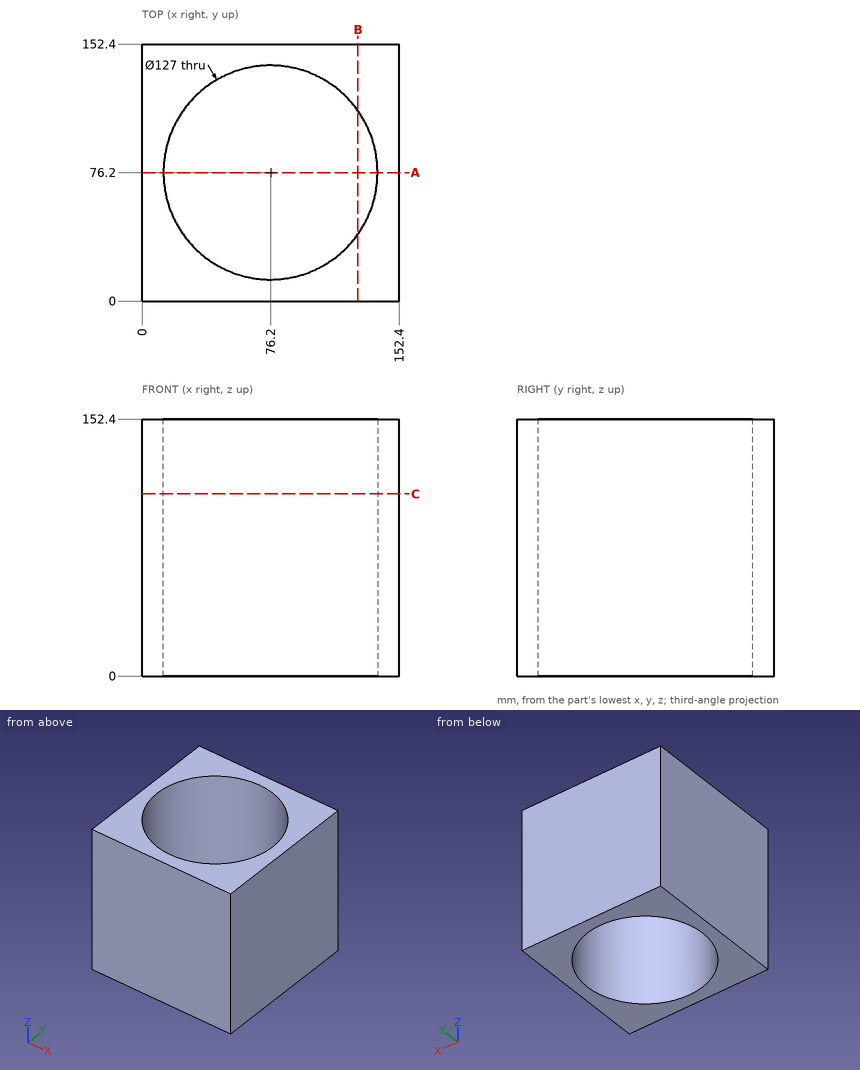
Design review of the part shown in the three views and the two pictorial views. Dimensions are in mm from the part's minimum x, y and z. Coordinates: 2 decimals unless noted, no trailing zeros. Loops run counter-clockwise (first coordinate to the right, second up) from the corner with the lowest first, then second, coordinate; pieces in that order, holes last. Notation, with made-up numbers: M -13.75,25 L 35.25,25 A22 ccw 35.25,37 Z; hole C 62.25,42.25 d7. An arc over 180 degrees is marked long. Put each result on its own line as item: value. Start each with the question number.
Q1. Add section B-B (x = 128). Write out the cut boundary in (y, z).
Q2. Wall thickness on line 1 (X direction, y = 76, z = 45); line 2 (Y direction, x = 130.5, z = 123.5): over which ranges is each line inside the solid? List them lowest first.
Q3. Add section A-A (y = 76.2). Write out the cut boundary in (x, z), and give its area (3 significant figures).
Q4. Add section C-C (z = 108). Write out the cut boundary in (x, y).
Answers:
1. outline: M 0,0 L 39.47,0 L 39.47,152.4 L 0,152.4 Z; M 112.93,0 L 152.4,0 L 152.4,152.4 L 112.93,152.4 Z
2. line 1: x = 0 to 12.7, 139.7 to 152.4
2. line 2: y = 0 to 43.28, 109.12 to 152.4
3. outline: M 0,0 L 12.7,0 L 12.7,152.4 L 0,152.4 Z; M 139.7,0 L 152.4,0 L 152.4,152.4 L 139.7,152.4 Z
3. area: 3,870 mm^2
4. outline: M 0,0 L 152.4,0 L 152.4,152.4 L 0,152.4 Z; hole C 76.2,76.2 d127
